Source: CAD feature listing. Evaluate the final solid. Frame: model axes, mm. Round coordinates to 2 decimals unless told otherwise and drop trailing zeros. Order: outer loops, then holes, each group sorted by start corner. A loop starts at its lowest first (then second) coordinate and runs counter-clockwise, first axis right, second up. Notation, with made-up numbers: (50, 59) - (97, 59) arc R10 cw to (97, 64) - close; hole circle Ø11 at (89, -17). An arc over 180 degrees is marked (long way). Return JSON: item names as keys, results as strings. Group by question number.
1) Section B-B, the plane z = -108.5. Return loops of the section in (x, y) (3 decimals), plus the area to 3 significant figures.
2) Section A-A, the plane y = 98. Return loops of the section in (x, z) (1 decimal), plus the area to 3 significant figures.
3) Section C-C, the plane x = 0.85. Give the number of separate pieces and of enclosed holes in the cut face, plus the area to 3 significant figures.
4) Ray query, line 1 (Y direction, x = 1.9, z = 32.5); line 2 (Y direction, x = 1.1, z = 0); line 3 (Z direction, x = 3.05, y = 17) (3 decimals). Return the intervals inside material, ascending. Write a range as from..to.
5) Contact query for flat-ended pins moving along their axis: P1, Ø0.7, axis at x = 2, z = 51, coming from the +Y side; P2, Ø1.8, axis at x = 2, z = 45, coming from the -Y side (3 decimals); P3, Ø1.6, axis at x = 2.5, y = 31, coming from the -Z side. Output: stop coordinate, or through.
6) Section D-D, the plane z = 17.5. Return loops of the section in (x, y) (3 decimals), plus the area to 3 significant figures.
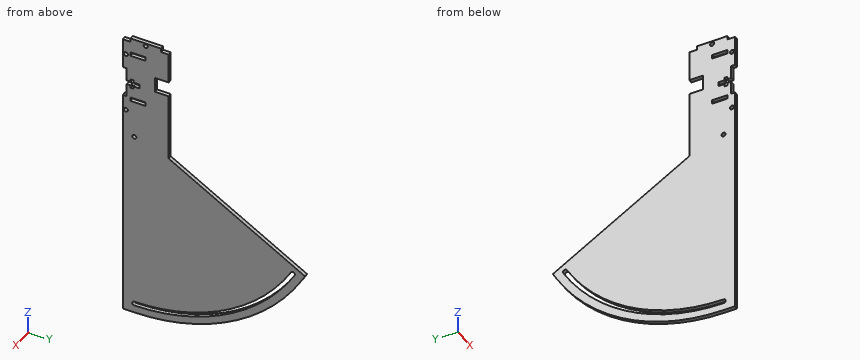
```python
from build123d import *

# Parameters (mm, degrees)
SKETCH1_R           = 1.7145
SKETCH1_W           = 3.175
SKETCH1_H           = 12.7
BOSS_EXTRUDE2_DEPTH = 3.175


with BuildPart() as part:
    # Sketch1 → Boss-Extrude2 (new body)
    with BuildSketch(Plane(origin=(0, 0, 0), x_dir=(0, 0, -1), z_dir=(1, 0, 0))):
        with BuildLine():
            Line((0, 0), (160.4645, 0))
            Line((160.4645, 0), (160.4645, 9.53262))
            ThreePointArc((160.4645, 9.53262), (138.966333406, 89.76487), (80.23225, 148.498953406))
            Line((80.23225, 148.498953406), (74.732988686, 151.673953406))
            Line((74.732988686, 151.673953406), (9.161036114, 38.1))
            Line((9.161036114, 38.1), (-47.625, 38.1))
            Line((-47.625, 38.1), (-47.625, 26.67))
            Line((-47.625, 26.67), (-60.325, 26.67))
            Line((-60.325, 26.67), (-60.325, 38.1))
            Line((-60.325, 38.1), (-85.725, 38.1))
            Line((-85.725, 38.1), (-85.725, 31.75))
            Line((-85.725, 31.75), (-88.9, 31.75))
            Line((-88.9, 31.75), (-88.9, 6.35))
            Line((-88.9, 6.35), (-85.725, 6.35))
            Line((-85.725, 6.35), (-85.725, 0))
            Line((-85.725, 0), (-60.325, 0))
            Line((-60.325, 0), (-60.325, 3.175))
            Line((-60.325, 3.175), (-49.3395, 3.175))
            Line((-49.3395, 3.175), (-49.3395, 6.35))
            Line((-49.3395, 6.35), (-51.562, 6.35))
            Line((-51.562, 6.35), (-51.562, 8.89))
            Line((-51.562, 8.89), (-49.3395, 8.89))
            Line((-49.3395, 8.89), (-49.3395, 13.97))
            Line((-49.3395, 13.97), (-45.9105, 13.97))
            Line((-45.9105, 13.97), (-45.9105, 8.89))
            Line((-45.9105, 8.89), (-43.688, 8.89))
            Line((-43.688, 8.89), (-43.688, 6.35))
            Line((-43.688, 6.35), (-45.9105, 6.35))
            Line((-45.9105, 6.35), (-45.9105, 3.175))
            Line((-45.9105, 3.175), (-34.925, 3.175))
            Line((-34.925, 3.175), (-34.925, 0))
            Line((-34.925, 0), (0, 0))
        make_face()
        with Locations((-86.36, 19.05)):
            Circle(SKETCH1_R, mode=Mode.SUBTRACT)
        with Locations((0, 9.53262)):
            Circle(SKETCH1_R, mode=Mode.SUBTRACT)
        with Locations((-73.025, 2.54)):
            Circle(SKETCH1_R, mode=Mode.SUBTRACT)
        with Locations((-22.225, 2.54)):
            Circle(SKETCH1_R, mode=Mode.SUBTRACT)
        with Locations((-74.6125, 12.7)):
            Rectangle(SKETCH1_W, SKETCH1_H, mode=Mode.SUBTRACT)
        with Locations((-33.3375, 12.7)):
            Rectangle(SKETCH1_W, SKETCH1_H, mode=Mode.SUBTRACT)
        with BuildLine():
            ThreePointArc((154.1145, 9.53262), (133.467072092, 86.58987), (77.05725, 142.999692092))
            ThreePointArc((77.05725, 142.999692092), (74.715199445, 142.372141537), (75.34275, 140.030090982))
            ThreePointArc((75.34275, 140.030090982), (130.497470982, 84.87537), (150.6855, 9.53262))
            ThreePointArc((150.6855, 9.53262), (152.4, 7.81812), (154.1145, 9.53262))
        make_face(mode=Mode.SUBTRACT)
    extrude(amount=BOSS_EXTRUDE2_DEPTH)


solid = part.part
```
Geometry check:
{
 "1": {"outline": "(0, 0) - (3.175, 0) - (3.175, 114.098) - (0, 114.098) - close; (0, 118.981) - (3.175, 118.981) - (3.175, 127.755) - (0, 127.755) - close", "area": "390 mm2"},
 "2": {"outline": "(0, -133.9) - (3.2, -133.9) - (3.2, -126.2) - (0, -126.2) - close; (0, -122) - (3.2, -122) - (3.2, -43.7) - (0, -43.7) - close", "area": "273 mm2"},
 "3": {"separate pieces": "1", "enclosed holes": "7", "area": "18,500 mm2"},
 "4": {"line 1": "0..6.35, 19.05..38.1", "line 2": "0..7.82, 11.25..38.1", "line 3": "-160.291..-153.933, -150.5..31.75, 34.925..73.025, 76.2..88.9"},
 "5": {"P1": "y = 26.67", "P2": "y = 3.175", "P3": "z = -159.13"},
 "6": {"outline": "(0, 0) - (3.175, 0) - (3.175, 38.1) - (0, 38.1) - close", "area": "121 mm2"}
}
